The listing builds one solid part. Answer for the finished solid, in the listing's coordinates (mm). Round coordinates to 2 decimals unless told otherwise and drop trailing zeros. Write each loop counter-clockwise with the first axis right and the second up, starting at its lowest first coordinate (ties: lowest second). Pieces come first, ordered by that corner, then holes.
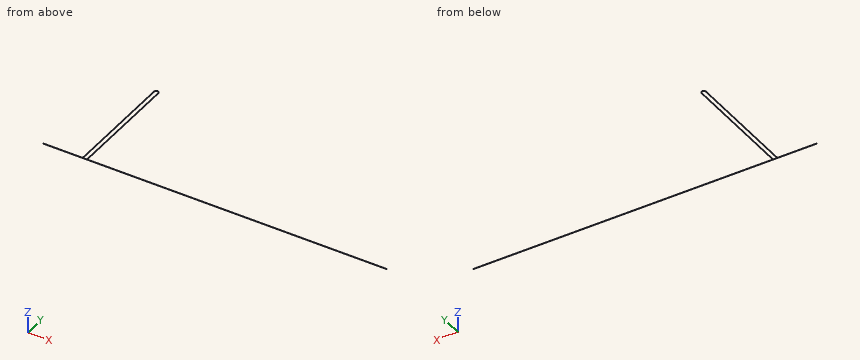
Autodesk Inventor part; units mm, degrees
ref_plane "YZ Plane" through (0, 0, 0) normal (1, 0, 0) x (0, 1, 0)
ref_plane "XZ Plane" through (0, 0, 0) normal (0, 1, 0) x (-1, 0, 0)
ref_plane "XY Plane" through (0, 0, 0) normal (0, 0, 1) x (1, 0, 0)
sketch "Sketch2" plane through (0, 0, 0) normal (0, 0, 1) x (1, 0, 0)
  line L0 (0, 0) -> (2420, 0)
  line L1 (2420, 0) -> (2420, 3)
  line L2 (2420, 3) -> (0, 3)
  line L3 (0, 3) -> (0, 0)
  line L4 (307, 3) -> (307, 803)
  line L5 (307, 803) -> (310, 803)
  line L6 (310, 803) -> (310, 3)
  line L7 (310, 803) -> (1110, 803) construction
  line L8 (277, 3) -> (277, 803)
  line L9 (277, 803) -> (280, 803)
  line L10 (280, 803) -> (280, 3)
  line L11 (310, 806) -> (310, 803)
  line L12 (310, 3) -> (307, 3)
  line L13 (277, 3) -> (280, 3)
  line L14 (277, 3) -> (280, 3)
  arc A0 (310, 803) -> (277, 803) centre (293.5, 803) ccw
  arc A1 (307, 803) -> (280, 803) centre (293.5, 803) ccw
  line L15 (277, 803) -> (280, 803)
  line L16 (307, 803) -> (310, 803)
  dimension "d16" = 2420
  dimension "d17" = 3
  dimension "d18" = 90
  dimension "d21" = 800
  dimension "d22" = 3
  dimension "d23" = 90
  dimension "d24" = 90
  dimension "d25" = 2110
  dimension "d28" = 30
extrude "Extrusion2" add sketch "Sketch2" along normal blind 6 contours L3 L2 L1 L0 | L8 L9 L10 L2 | L2 L4 L5 L6 | A0 L5 A1 L9
properties part number "BeltMain" material "Rubber"
1. Section A-A on y = 693.5 is taken. Determine the outline of the cut face in (x, z), plus the area to 3 significant figures.
Geometry says:
outline: (277, 0) - (280, 0) - (280, 6) - (277, 6) - close; (307, 0) - (310, 0) - (310, 6) - (307, 6) - close
area: 36.0 mm2
2. Straight lines are drawn through the part: line 1 along X through (y, z) = (627, 1.6); line 2 along Y through (x, z) = (335, 1.6); line 3 along Y through (x, z) = (301.5, 2.3). For each, find the intervals that lie inside material, in ascending order.
Geometry says:
line 1: x = 277 to 280, 307 to 310
line 2: y = 0 to 3
line 3: y = 0 to 3, 813.87 to 817.43
3. Given pin 1 (1.5 mm diameter, centred on y = 432.5, z = 2.5, fed in from +X); pin 2 (1 mm diameter, centred on y = 401, z = 1, fed in from -X); pin 3 (3 mm diameter, centred on x = 172, z = 3, fed in from +Y); pin 4 (3 mm diameter, centred on x = 292.5, z = 3.5, fed in from +Y), each flat-ended and moving along its own axis, determine where each tip first touches the part or whether it passes through.
Geometry says:
pin 1: stops at x = 310
pin 2: stops at x = 277
pin 3: stops at y = 3
pin 4: stops at y = 819.5
4. Section B-B on z = 4.2 is taken. Determine the outline of the cut face in (x, y).
Geometry says:
outline: (0, 0) - (2420, 0) - (2420, 3) - (310, 3) - (310, 803) arc R16.5 ccw to (277, 803) - (277, 3) - (0, 3) - close; hole (280, 3) - (307, 3) - (307, 803) arc R13.5 ccw to (280, 803) - close
5. Section C-C on x = 941 is taken. Determine the outline of the cut face in (y, z).
Geometry says:
outline: (0, 0) - (3, 0) - (3, 6) - (0, 6) - close
